Part model, mm, in its own coordinate system. Round coordinates to 2 decimals unless told otherwise and drop trailing zeros. Loops run counter-clockwise (first coordinate to the right, second up) from the corner with the lowest first, then second, coordinate; pieces in that order, holes last.
1) Probe line 1 (X direction, y = 61, z = 1.1); line 2 (X direction, y = 11, z = 1.4); line 3 (Y direction, x = -1, z = 2.2). List the from-to ranges inside material, lowest first.
2) Drop flat-ended pins along their axis: P1, Ø1.5, axis at y = 15.5, z = -0.5, coming from the +X side; P2, Ø1.5, axis at x = -21.5, z = 0, coming from the +Y side; P3, Ø1, axis at y = -21.5, z = -0.5, coming from the -X side; P4, Ø10.5, axis at x = 0, y = -29, coming from the -Z side. Give the stop position or say it passes through.
3) Band-saw the part on B-B, the plane x = 0. Write the cut outline in (y, z), then the cut area to 3 significant figures.
4) Band-saw the part on A-A, the plane y = 41. Write the cut outline in (x, z), then the cut area to 3 significant figures.
5) Band-saw the part on C-C, the plane z = -1.05. State how many separate pieces and enclosed holes the cut face has, then the cut area to 3 significant figures.
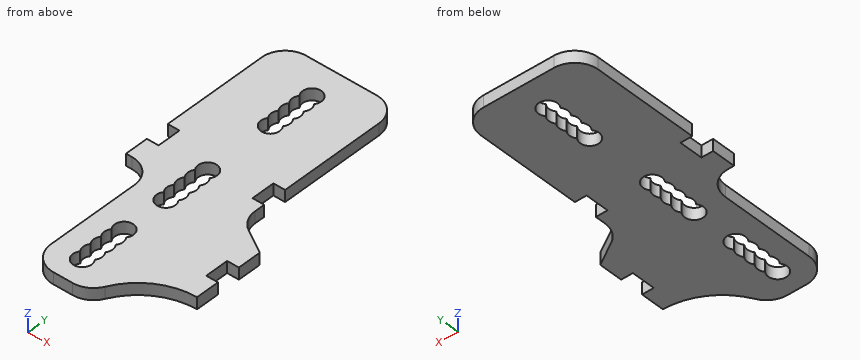
from build123d import *

# Parameters (mm, degrees)
BOSS_EXTRUDE1_DEPTH = 2.5
FILLET1_R           = 10


with BuildPart() as part:
    # Sketch1 → Boss-Extrude1 (new, symmetric)
    with BuildSketch(Plane(origin=(0, 0, 0), x_dir=(0, 1, 0), z_dir=(0, 0, 1))):
        with BuildLine():
            Line((10, 25), (0, 25))
            Line((0, 25), (0, 12.5))
            Line((0, 12.5), (-60, 12.5))
            Line((-60, 12.5), (-60, -12.5))
            ThreePointArc((-60, -12.5), (-44.850338923, -22.699349723), (-39, -40))
            Line((-39, -40), (-29, -40))
            Line((-29, -40), (-29, -35))
            Line((-29, -35), (-19, -35))
            Line((-19, -35), (-19, -40))
            Line((-19, -40), (-9, -40))
            Line((-9, -40), (0, -25))
            Line((0, -25), (10, -25))
            Line((10, -25), (10, -20))
            Line((10, -20), (20, -20))
            Line((20, -20), (20, -25))
            Line((20, -25), (75, -25))
            Line((75, -25), (75, 25))
            Line((75, 25), (20, 25))
            Line((20, 25), (20, 20))
            Line((20, 20), (10, 20))
            Line((10, 20), (10, 25))
        make_face()
        with BuildLine():
            ThreePointArc((-46.5, 3.122498999), (-44, 4), (-41.5, 3.122498999))
            ThreePointArc((-41.5, 3.122498999), (-39, 4), (-36.5, 3.122498999))
            ThreePointArc((-36.5, 3.122498999), (-34, 4), (-31.5, 3.122498999))
            ThreePointArc((-31.5, 3.122498999), (-27.267949192, 3.605551275), (-25, 0))
            ThreePointArc((-25, 0), (-27.267949192, -3.605551275), (-31.5, -3.122498999))
            ThreePointArc((-31.5, -3.122498999), (-34, -4), (-36.5, -3.122498999))
            ThreePointArc((-36.5, -3.122498999), (-39, -4), (-41.5, -3.122498999))
            ThreePointArc((-41.5, -3.122498999), (-44, -4), (-46.5, -3.122498999))
            ThreePointArc((-46.5, -3.122498999), (-53, 0), (-46.5, 3.122498999))
        make_face(mode=Mode.SUBTRACT)
        with BuildLine():
            ThreePointArc((-6.5, 3.122498999), (-4, 4), (-1.5, 3.122498999))
            ThreePointArc((-1.5, 3.122498999), (1, 4), (3.5, 3.122498999))
            ThreePointArc((3.5, 3.122498999), (6, 4), (8.5, 3.122498999))
            ThreePointArc((8.5, 3.122498999), (12.732050808, 3.605551275), (15, 0))
            ThreePointArc((15, 0), (12.732050808, -3.605551275), (8.5, -3.122498999))
            ThreePointArc((8.5, -3.122498999), (6, -4), (3.5, -3.122498999))
            ThreePointArc((3.5, -3.122498999), (1, -4), (-1.5, -3.122498999))
            ThreePointArc((-1.5, -3.122498999), (-4, -4), (-6.5, -3.122498999))
            ThreePointArc((-6.5, -3.122498999), (-13, 0), (-6.5, 3.122498999))
        make_face(mode=Mode.SUBTRACT)
        with BuildLine():
            ThreePointArc((43.5, 3.122498999), (46, 4), (48.5, 3.122498999))
            ThreePointArc((48.5, 3.122498999), (51, 4), (53.5, 3.122498999))
            ThreePointArc((53.5, 3.122498999), (56, 4), (58.5, 3.122498999))
            ThreePointArc((58.5, 3.122498999), (62.732050808, 3.605551275), (65, 0))
            ThreePointArc((65, 0), (62.732050808, -3.605551275), (58.5, -3.122498999))
            ThreePointArc((58.5, -3.122498999), (56, -4), (53.5, -3.122498999))
            ThreePointArc((53.5, -3.122498999), (51, -4), (48.5, -3.122498999))
            ThreePointArc((48.5, -3.122498999), (46, -4), (43.5, -3.122498999))
            ThreePointArc((43.5, -3.122498999), (37, 0), (43.5, 3.122498999))
        make_face(mode=Mode.SUBTRACT)
    extrude(amount=BOSS_EXTRUDE1_DEPTH, both=True)

    # Fillet1
    fillet1_edges = [part.edges().sort_by_distance(p)[0] for p in [
        (-12.5, -60, 0),
        (-12.5, 0, 0),
        (-25, 75, 0),
        (25, 75, 0),
        (25, 0, 0),
        (12.5, -60, 0),
    ]]
    fillet(fillet1_edges, radius=FILLET1_R)


solid = part.part
Reported:
1. line 1: x = -25 to -4, 4 to 25
1. line 2: x = -20 to -4, 4 to 20
1. line 3: y = -60 to -52.87, -25.13 to -12.87, 14.87 to 37.13, 64.87 to 75
2. P1: stops at x = 20
2. P2: stops at y = 73.18
2. P3: stops at x = -12.5
2. P4: stops at z = -2.5
3. outline: (-60, -2.5) - (-53, -2.5) - (-53, 2.5) - (-60, 2.5) - close; (-25, -2.5) - (-13, -2.5) - (-13, 2.5) - (-25, 2.5) - close; (15, -2.5) - (37, -2.5) - (37, 2.5) - (15, 2.5) - close; (65, -2.5) - (75, -2.5) - (75, 2.5) - (65, 2.5) - close
3. area: 255 mm2
4. outline: (-25, -2.5) - (-4, -2.5) - (-4, 2.5) - (-25, 2.5) - close; (4, -2.5) - (25, -2.5) - (25, 2.5) - (4, 2.5) - close
4. area: 210 mm2
5. separate pieces: 1
5. enclosed holes: 3
5. area: 5,610 mm2
